CAD build for the part. Positions are in the model's coordinates, mm. Face numbers are marked on the shaded views. Coordinates: 2 decimals unless noted, no trailing zeros. Write each loop counter-clockwise with the first axis right and the second up, starting at its lowest first coordinate (ties: lowest second). Pieces come first, ordered by that corner, then holes. Notation, with made-up numbers: M 86,31 L 93,31 A28 ccw 93,67 Z; hole C 18.5,-17.75 d6. An arc over 180 degrees is marked long. Answer as CSV lines item,"result". Start each with the question number.
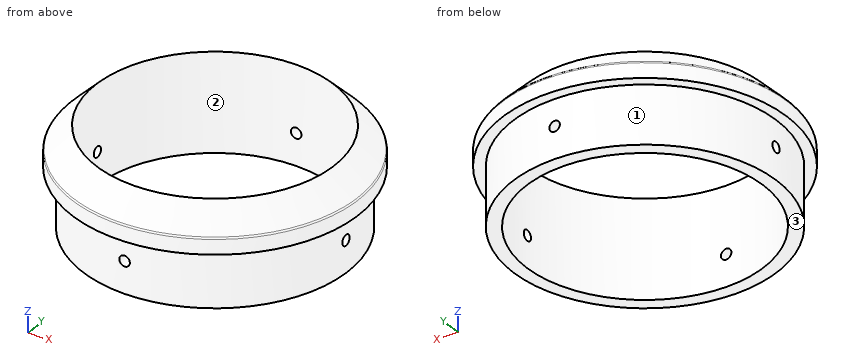
```python
from build123d import *

# Parameters (mm, degrees)
F0_R           = 27
F1_DEPTH       = 8
F2_SIZE        = 5
F3_R           = 0.5
F4_R           = 25
F5_DEPTH       = 11
F6_R           = 22.45
F7_DEPTH       = 19.001
F8_R           = 1
F9_DEPTH       = 27.0010008385
F9_DEPTH_BACK  = 27.0010008385
F10_R          = 1
F11_DEPTH      = 27.0010001
F11_DEPTH_BACK = 27.0010001


with BuildPart() as f1:
    # F0 (on Top) → F1 (new body)
    with BuildSketch(Plane.XY):
        Circle(F0_R)
    extrude(amount=F1_DEPTH)

    # F2
    f2_edges = [f1.edges().sort_by_distance(p)[0] for p in [
        (-27, 0, 8),
    ]]
    chamfer(f2_edges, length=F2_SIZE)

    # F3
    f3_edges = [f1.edges().sort_by_distance(p)[0] for p in [
        (-22, 0, 8),
        (-27, 0, 3),
    ]]
    fillet(f3_edges, radius=F3_R)

    # F4 (on face) → F5 (join)
    with BuildSketch(Plane(origin=(0, 0, 0), x_dir=(1, 0, 0), z_dir=(0, 0, -1))):
        Circle(F4_R)
    extrude(amount=F5_DEPTH)

    # F6 (on face) → F7 (cut, through all)
    with BuildSketch(Plane.XY.offset(8)):
        Circle(F6_R)
    extrude(amount=-F7_DEPTH, mode=Mode.SUBTRACT)

    # F8 (on Front) → F9 (cut, two sides)
    with BuildSketch(Plane.XZ) as f9_sk:
        with Locations((0, -5)):
            Circle(F8_R)
    extrude(amount=-F9_DEPTH, mode=Mode.SUBTRACT)
    extrude(f9_sk.sketch, amount=F9_DEPTH_BACK, mode=Mode.SUBTRACT)

    # F10 (on Right) → F11 (cut, two sides)
    with BuildSketch(Plane.YZ) as f11_sk:
        with Locations((0, -5)):
            Circle(F10_R)
    extrude(amount=F11_DEPTH, mode=Mode.SUBTRACT)
    extrude(f11_sk.sketch, amount=-F11_DEPTH_BACK, mode=Mode.SUBTRACT)


solid = f1.part
```
1) Band-saw the part on A-A, the plane z = -5. List the corners of the cut face in (x, y).
2) Band-saw the part on D-D, the plane z = -1.75. List the corners of the cut face in (x, y).
3) Probe L1, parallel to Y at x = 0.5, z = -3 (3 decimals); L2, parallel to X at y = 0, z = -2; L3, parallel to X at y = -6, z = -6.75. List the from-to ranges inside material, lowest first. Write a range as [from, to].
4) Two-plate mould, pull along X, no slides. Class the marked faces 1, 2 and 3: pulls with the +X half, pulls with the -X half, needs draft (parallel to the pull), parting line crosses it, or undercut.
5) Pin check, flat tips, straight feed: P1, Ø10, axis at x = 11.5, z = 1, coming from the -Y side; P2, Ø1, axis at y = 19, z = 4.5, coming from the +X side; P3, Ø5, axis at x = 16, z = -1.5, coming from the +Y side. Stop position of each tip, or through.
6) Band-saw the part on B-B, the plane x = 0. State how many separate pieces and enclosed holes the cut face has, plus the area to 3 significant figures.
Result sheet:
1,outline,"M -24.98,-1 A25 ccw -1,-24.98 L -1,-22.43 A22.45 cw -22.43,-1 Z; M -24.98,1 L -22.43,1 A22.45 cw -1,22.43 L -1,24.98 A25 ccw Z; M 1,-24.98 A25 ccw 24.98,-1 L 22.43,-1 A22.45 cw 1,-22.43 Z; M 1,22.43 A22.45 cw 22.43,1 L 24.98,1 A25 ccw 1,24.98 Z"
2,outline,"C 0,0 d50; hole C 0,0 d44.9"
3,L1,"y = [-24.995, -22.444], [22.444, 24.995]"
3,L2,"x = [-25, -22.45], [22.45, 25]"
3,L3,"x = [-24.27, -21.63], [21.63, 24.27]"
4,face 1,"parting line crosses it"
4,face 2,"undercut"
4,face 3,"needs draft"
5,P1,"stops at y = -26.21"
5,P2,"stops at x = 17.92"
5,P3,"stops at y = 23.09"
6,separate pieces,"4"
6,enclosed holes,"0"
6,area,"93.9 mm²"
